Design review of the part built by this model. Coordinates are the model's own, in mm. A direction names the side the tool comes from. Coordinates: 2 decimals unless noted, no trailing zeros. Loops run counter-clockwise (first coordinate to the right, second up) from the corner with the lowest first, then second, coordinate; pieces in that order, holes last. Notation, with made-up numbers: M 40,38.5 L 77,38.5 A36 cw 77,76.5 Z; hole C 84.5,79.25 d8. An arc over 180 degrees is marked long. Put each result on its own line as item: value. Start each with the question number.
(1) The part is to be moulded in two halves that separate along Z. For faces 5 (the flat face through (32.024, 0.852, 47.821)), 6 (the conical face through (-2.3, 7.2, 92.2)), 7 (the flat face through (-20.18, -29, 22.14)), say which applies: +Z half, -Z half, draft (parallel to the pull), parting line (faces both ways), or undercut.
(2) Take a section at C-C, the plane z = 82. Give the boundary of the cut face in (x, y), then the cut area to 3 significant figures.
(3) For faces 1 (the flat face through (-18, 30, 66)), 2 (the flat face through (-13.417, -30.59, 17.871)), 3 (the flat face through (-21.034, 31.365, 32.538)), 4 (the flat face through (1, 1, 0)), list the 3-axis set-ups (+Z, -Z, +X, -X, +Y, -Y) from which the entire face can be reached by the end or side of a thin tool; tool diameter is ignored.
(4) For probe 1 along Z at (x, y) = (-17, 28.5); probe 2 along Y at (x, z) = (2.5, 5.5); probe 3 along X at (y, z) = (29, 52), list the stretches that pass through material, from the lowest coordinate up. Write a range as [from, to].
(5) Take a section at B-B, the plane y = -30. Give the boundary of the cut face in (x, z).
(6) Clearance check with flat-ended pins moving along their axes: pin 1 (15.5 mm diameter, centred on x = -17, y = 30.5, fed in from +Z); pin 2 (1 mm diameter, centred on y = -31, z = 47, fed in from -X); pin 3 (5 mm diameter, centred on x = 36.5, z = 14, fed in from +Y). State where each tip first meets the part, or that it passes through.
(7) Take a section at A-A, the plane z = 55.5. Give the boundary of the cut face in (x, y).
```python
from build123d import *

# Parameters (mm, degrees)
F3_DEPTH = 66
F5_DEPTH = 25
F7_DEPTH = 25


with BuildPart() as f1:
    # F0 (on Right) → F1 (revolve)
    with BuildSketch(Plane.YZ):
        Polygon((27.9374904931, 66.2788972259), (0, 101.8101840481), (0, 0), (27.9374904931, 0), align=None)
    revolve(axis=Axis((0, 0, 50.905092024), (0, 0, 1)))

    # F2 (on Top) → F3 (join)
    with BuildSketch(Plane.XY):
        Polygon((47.6167220591, 0), (27.1738618612, 5.2120122127), (27.5337807834, -4.8169167712), align=None)
        Polygon((-9.5953180999, 26.2534120063), (-23.8083610295, 41.2372909481), (-18.1006659117, 20.9272485844), align=None)
        Polygon((-17.9384626835, -21.4364952351), (-23.8083610295, -41.2372909481), (-9.0731959496, -26.1392607971), align=None)
    extrude(amount=F3_DEPTH)

    # F4 (on face) → F5 (cut)
    with BuildSketch(Plane(origin=(2.5903057561, -10.7996382035, 0), x_dir=(0.9724201368, 0.2332360983, 0), z_dir=(0.2332360983, -0.9724201368, 0))):
        Polygon((46.3034593785, 66), (25.6509240024, 66), (46.3034593785, 0), align=None)
    extrude(amount=-F5_DEPTH, mode=Mode.SUBTRACT)

    # F6 (on face) → F7 (cut)
    with BuildSketch(Plane(origin=(8.4188237579, -8.2164862973, 0), x_dir=(0.6984544852, 0.7156544782, 0), z_dir=(0.7156544782, -0.6984544852, 0))):
        Polygon((-46.1407084808, 66), (-46.1407084808, 0), (-25.3400105467, 66), align=None)
    extrude(amount=-F7_DEPTH, mode=Mode.SUBTRACT)


solid = f1.part
```
Computed values:
1. face 5: undercut
1. face 6: +Z half
1. face 7: draft
2. outline: C 0,0 d31.15
2. area: 762 mm^2
3. face 1: +Z, -X, +Y
3. face 2: +Z, -Z, -Y
3. face 3: +Z, -Z, -X
3. face 4: -Z, +X, -X, +Y, -Y
4. probe 1: z = [0, 66]
4. probe 2: y = [-27.83, 27.83]
4. probe 3: x = [-20.37, -12.2]
5. outline: M -20.48,0 L -12.84,0 L -12.84,49.82 L -20.48,32.9 Z
6. pin 1: stops at z = 67.26
6. pin 2: stops at x = -13.65
6. pin 3: stops at y = 3.47
7. outline: M -23.81,41.24 L -18.18,21.21 A27.94 ccw -17.88,-21.47 L -17.94,-21.44 L -18.19,-22.28 L -11.59,-28.72 L -9.28,-26.35 A27.94 ccw 27.53,-4.75 L 27.53,-4.82 L 30.73,-4.05 L 28.59,4.85 L 27.46,5.14 A27.94 ccw -9.65,26.22 L -9.6,26.25 Z
